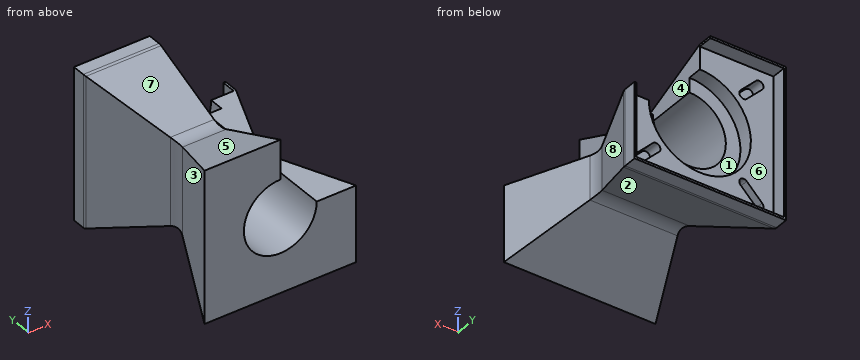
from build123d import *

# Parameters (mm, degrees)
SKETCH1_W               = 104
SKETCH1_H               = 104
BOSS_EXTRUDE1_DEPTH     = 125
CUT_EXTRUDE3_DEPTH      = 125
CUT_EXTRUDE4_DEPTH      = 146.027583583
CUT_EXTRUDE4_DEPTH_BACK = 146.027583583
CUT_EXTRUDE5_DEPTH      = 146.027583583
CUT_EXTRUDE5_DEPTH_BACK = 146.027583583
SKETCH4_R               = 25
SKETCH5_W               = 101
SKETCH5_H               = 101
CUT_EXTRUDE6_DEPTH      = 10
SKETCH6_W               = 52
SKETCH6_H               = 52
CUT_EXTRUDE7_DEPTH      = 125
SKETCH7_W               = 52
SKETCH7_H               = 52
CUT_EXTRUDE8_DEPTH      = 125
SKETCH8_R               = 35
CUT_EXTRUDE9_DEPTH      = 10
CUT_EXTRUDE10_DEPTH     = 10
FILLET3_R               = 5
FILLET4_R               = 15


with BuildPart() as part:
    # Sketch1 → Boss-Extrude1 (new body)
    with BuildSketch(Plane(origin=(0, 0, 0), x_dir=(1, 0, 0), z_dir=(0, 1, 0))):
        Rectangle(SKETCH1_W, SKETCH1_H)
    extrude(amount=BOSS_EXTRUDE1_DEPTH)

    # Sketch2 → Cut-Extrude3 (cut)
    with BuildSketch(Plane.XY.offset(52)):
        Polygon((-27.592698068, 57.5), (-52, 115), (-52, 0), align=None)
        Polygon((52, 0), (52, 115), (27.592698068, 57.5), align=None)
    extrude(amount=-CUT_EXTRUDE3_DEPTH, mode=Mode.SUBTRACT)

    # Sketch3 → Cut-Extrude4 (cut, two sides: drawn at the far end of the back side and taken through both)
    with BuildSketch(Plane(origin=(0, 0, 0), x_dir=(0, 0, -1), z_dir=(1, 0, 0)).offset(-CUT_EXTRUDE4_DEPTH_BACK)):
        Polygon((-52, 115), (-27.592698068, 57.5), (-52, 0), align=None)
        Polygon((52, 115), (27.592698068, 57.5), (52, 0), align=None)
    extrude(amount=CUT_EXTRUDE4_DEPTH + CUT_EXTRUDE4_DEPTH_BACK, mode=Mode.SUBTRACT)

    # Sketch4 → Cut-Extrude5 (cut, two sides: drawn at the far end of the back side and taken through both)
    with BuildSketch(Plane(origin=(0, 125, 0), x_dir=(1, 0, 0), z_dir=(0, 1, 0)).offset(-CUT_EXTRUDE5_DEPTH_BACK)):
        with Locations(Location((0, 0, 0), (0, 0, 270))):
            Circle(SKETCH4_R)
    extrude(amount=CUT_EXTRUDE5_DEPTH + CUT_EXTRUDE5_DEPTH_BACK, mode=Mode.SUBTRACT)

    # Sketch5 → Cut-Extrude6 (cut)
    with BuildSketch(Plane(origin=(0, 125, 0), x_dir=(1, 0, 0), z_dir=(0, 1, 0))):
        Rectangle(SKETCH5_W, SKETCH5_H)
    extrude(amount=-CUT_EXTRUDE6_DEPTH, mode=Mode.SUBTRACT)

    # Sketch6 → Cut-Extrude7 (cut)
    with BuildSketch(Plane(origin=(0, 115, 0), x_dir=(1, 0, 0), z_dir=(0, 1, 0))):
        with Locations((26, -26)):
            Rectangle(SKETCH6_W, SKETCH6_H)
    extrude(amount=-CUT_EXTRUDE7_DEPTH, mode=Mode.SUBTRACT)

    # Sketch7 → Cut-Extrude8 (cut)
    with BuildSketch(Plane(origin=(0, 125, 0), x_dir=(1, 0, 0), z_dir=(0, 1, 0))):
        with Locations((26, -26)):
            Rectangle(SKETCH7_W, SKETCH7_H)
    extrude(amount=-CUT_EXTRUDE8_DEPTH, mode=Mode.SUBTRACT)

    # Sketch8 → Cut-Extrude9 (cut)
    with BuildSketch(Plane(origin=(0, 115, 0), x_dir=(1, 0, 0), z_dir=(0, 1, 0))):
        Circle(SKETCH8_R)
    extrude(amount=-CUT_EXTRUDE9_DEPTH, mode=Mode.SUBTRACT)

    # Sketch9 → Cut-Extrude10 (cut)
    with BuildSketch(Plane(origin=(0, 115, 0), x_dir=(1, 0, 0), z_dir=(0, 1, 0))):
        with BuildLine():
            Line((-38.537319575, 42.779960262), (-27.930717857, 32.173358544))
            ThreePointArc((-27.930717857, 32.173358544), (-27.930717857, 27.930717857), (-32.173358544, 27.930717857))
            Line((-32.173358544, 27.930717857), (-42.779960262, 38.537319575))
            ThreePointArc((-42.779960262, 38.537319575), (-42.779960262, 42.779960262), (-38.537319575, 42.779960262))
        make_face()
        with BuildLine():
            Line((38.537319575, 42.779960262), (27.930717857, 32.173358544))
            ThreePointArc((27.930717857, 32.173358544), (27.930717857, 27.930717857), (32.173358544, 27.930717857))
            Line((32.173358544, 27.930717857), (42.779960262, 38.537319575))
            ThreePointArc((42.779960262, 38.537319575), (42.779960262, 42.779960262), (38.537319575, 42.779960262))
        make_face()
        with BuildLine():
            Line((-38.537319575, -42.779960262), (-27.930717857, -32.173358544))
            ThreePointArc((-27.930717857, -32.173358544), (-27.930717857, -27.930717857), (-32.173358544, -27.930717857))
            Line((-32.173358544, -27.930717857), (-42.779960262, -38.537319575))
            ThreePointArc((-42.779960262, -38.537319575), (-42.779960262, -42.779960262), (-38.537319575, -42.779960262))
        make_face()
    extrude(amount=-CUT_EXTRUDE10_DEPTH, mode=Mode.SUBTRACT)

    # Fillet3
    fillet3_edges = [part.edges().sort_by_distance(p)[0] for p in [
        (-52, 115, 0),
        (52, 115, -26),
        (-26, 115, 52),
        (0, 115, -52),
    ]]
    fillet(fillet3_edges, radius=FILLET3_R)

    # Fillet4
    fillet4_edges = [part.edges().sort_by_distance(p)[0] for p in [
        (-27.592698068, 57.5, 0),
        (27.592698068, 57.5, -13.796349034),
        (-13.796349034, 57.5, 27.592698068),
        (0, 57.5, -27.592698068),
    ]]
    fillet(fillet4_edges, radius=FILLET4_R)


solid = part.part
Model file for the job. Use its own axes, mm. Face numbers are marked on the shaded views. A direction names the side the tool comes from. Round coordinates to 2 decimals unless told otherwise and drop trailing zeros. Order: outer loops, then holes, each group sorted by start corner. A loop starts at its lowest first (then second) coordinate and runs counter-clockwise, first axis right, second up.
(1) Band-saw the part on C-C (z = 9). List the corners of the cut face in (x, y).
(2) Drill centre lines: line 1 (Z direction, x = -18, y = 116); line 2 (Y direction, x = -42, z = 25); line 3 (Z direction, x = -8.5, y = 11.5). Where is each one in solid material? Low to high.
(3) Pin check, flat tips, straight feed: pin 1 (1 mm diameter, centred on y = 84.5, z = -36.5, fed in from +X); pin 2 (10 mm diameter, centred on y = 49, z = -39, fed in from +X); pin 3 (1.5 mm diameter, centred on y = 33.5, z = -3.5, fed in from +X); pin 4 (21.5 mm diameter, centred on y = 41, z = 43.5, fed in from +X). Stop position of each tip, or through.
(4) Pull direction Z, two halves, no side cores. Call the marked faces 6, 7 and 8: released by +Z, released by -Z, zero draft, split by the parting line, or undercut.
(5) Band-saw the part on A-A (z = -23). List the corners of the cut face in (x, y), then the cut area to 3 significant figures.
(6) 3-axis set-ups, long thin cutter, end or side, ignore diameter. For the marked faces 1, 2, 3, 4 and 5: which of +Z, -Z, +X, -X, +Y, -Y reach the whole face in a straight line?
(7) Band-saw the part on B-B (x = -11). List the corners of the cut face in (y, z), then the cut area to 3 significant figures.
(8) Band-saw the part on D-D (y = 99). List the corners of the cut face in (x, z), then the cut area to 3 significant figures.
Verdict:
1. outline: (-52, 0) - (-23.32, 0) - (-23.32, 105) - (-33.82, 105) - (-33.82, 115) - (-50.5, 115) - (-50.5, 125) - (-52, 125) - (-52, 116.02) arc R5 ccw to (-51.6, 114.06) - (-30.08, 63.36) arc R15 cw to (-30.08, 51.64) - close
2. line 1: z = -52 to -50.5, 50.5 to 52
2. line 2: y = 0 to 23.56, 91.44 to 115
2. line 3: z = -47.12 to -23.51, 23.51 to 47.12
3. pin 1: stops at x = 39.27
3. pin 2: passes through
3. pin 3: stops at x = 38.1
3. pin 4: stops at x = 0
4. face 6: undercut
4. face 7: released by +Z
4. face 8: zero draft
5. outline: (-52, 0) - (-9.8, 0) - (-9.8, 105) - (-26.38, 105) - (-26.38, 115) - (-50.5, 115) - (-50.5, 125) - (-52, 125) - (-52, 116.02) arc R5 ccw to (-51.6, 114.06) - (-30.08, 63.36) arc R15 cw to (-30.08, 51.64) - close; (9.8, 0) - (52, 0) - (30.08, 51.64) arc R15 cw to (30.08, 63.36) - (51.6, 114.06) arc R5 ccw to (52, 116.02) - (52, 125) - (50.5, 125) - (50.5, 115) - (26.38, 115) - (26.38, 105) - (9.8, 105) - close
5. area: 6,610 mm2
6. face 1: +Y
6. face 2: -Z, +X, -X
6. face 3: +Z, -Z, -X
6. face 4: +Z, +X, +Y, -Y
6. face 5: +Z, +X, -X
7. outline: (0, -52) - (51.64, -30.08) arc R15 cw to (63.36, -30.08) - (114.06, -51.6) arc R5 ccw to (116.02, -52) - (125, -52) - (125, -50.5) - (115, -50.5) - (115, -33.23) - (105, -33.23) - (105, -22.45) - (0, -22.45) - close; (0, 22.45) - (105, 22.45) - (105, 33.23) - (115, 33.23) - (115, 50.5) - (125, 50.5) - (125, 52) - (116.02, 52) arc R5 ccw to (114.06, 51.6) - (63.36, 30.08) arc R15 cw to (51.64, 30.08) - (0, 52) - close
7. area: 3,810 mm2
8. outline: (-45.21, -45.21) - (45.21, -45.21) - (45.21, 0) - (25, 0) arc R25 cw (long way) to (0, 25) - (0, 45.21) - (-45.21, 45.21) - close
8. area: 4,660 mm2
